```python
from build123d import *

# Parameters (mm, degrees)
CUT_EXTRUDE1_START = -2.5
CUT_EXTRUDE1_DEPTH = 2.5
SKETCH4_R          = 2.309401077
CUT_EXTRUDE2_DEPTH = 0.5
CUT_EXTRUDE2_TAPER = 45


with BuildPart() as part:
    # Sketch2 → Revolve1 (revolve)
    with BuildSketch(Plane(origin=(0, 0, 0), x_dir=(0, 0, -1), z_dir=(1, 0, 0))):
        Polygon((-9.25, 4.25), (-4.75, 4.25), (-4.5, 4), (-4.5, 2.5), (8.7, 2.5), (9.5, 1.7), (9.5, 0), (-9.5, 0), (-9.5, 4), align=None)
    revolve(axis=Axis((0, 0, -9.5), (0, 0, 1)))

    # Sketch3 → Cut-Extrude1 (cut)
    with BuildSketch(Plane.XY.offset(9.5).offset(CUT_EXTRUDE1_START)):
        Polygon((0, 2.309401077), (-2, 1.154700538), (-2, -1.154700538), (0, -2.309401077), (2, -1.154700538), (2, 1.154700538), align=None)
    extrude(amount=CUT_EXTRUDE1_DEPTH, mode=Mode.SUBTRACT)

    # Sketch4 → Cut-Extrude2 (cut)
    with BuildSketch(Plane.XY.offset(9.5)):
        Circle(SKETCH4_R)
    extrude(amount=-CUT_EXTRUDE2_DEPTH, taper=CUT_EXTRUDE2_TAPER, mode=Mode.SUBTRACT)


solid = part.part
```
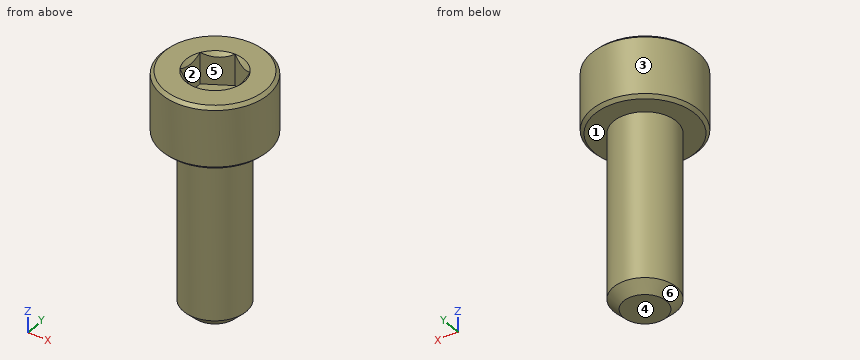
Part model, mm, in its own coordinate system. Face numbers are marked on the shaded views. A direction names the side the tool comes from. Give positions to 0.01 mm unless a question says otherwise; leave off trailing zeros. Order: outer loops, then holes, each group sorted by start corner. A loop starts at its lowest first (then second) coordinate and runs counter-clockwise, first axis right, second up. Notation, with made-up numbers: M -38,35.5 L -7,35.5 A33 ccw -7,74.5 Z; hole C 3,-36.75 d6. An arc over 180 degrees is marked long. Use a Markdown table: item, result. Add a question column.
(1) Probe line 1 along Z through (x, y) = (-1.25, -2.25); line 2 along X through (y, z) = (1.5, -4.75); line 3 along Z through (x, y) = (-1.5, -0.5). List the from-to ranges inside material, lowest first. Write a range as [from, to].
(2) Drop flat-ended pins along their axis: P1, Ø1.5, axis at x = 1.5, y = -1.5, coming from the +Z side; P2, Ø1, axis at x = 2.5, z = 5.5, coming from the -Y side; P3, Ø1.2, axis at x = -1, y = 0, coming from the +Z side; P4, Ø1, axis at y = -2.5, z = 5.5, coming from the +X side. Give the stop position or say it passes through.
(3) Saw through at A-A, the plane y = 0. Give the cut face in (x, z), and give its area (3 significant figures).
(4) 3-axis set-ups, long thin cutter, end or side, ignore diameter. For the marked faces 1, 2 and 3: which of +Z, -Z, +X, -X, +Y, -Y reach the whole face in a straight line?
(5) Saw through at C-C, the plane z = 5.5. Give the cut face in (x, y).
(6) Saw through at B-B, the plane z = -8. Give the cut face in (x, y).
(7) Mould opens along Y. For the marked faces 4, 5 and 6 say: +Y half, -Y half, draft (parallel to the pull), parting line (faces both ways), or undercut.
Answer key:
| question | item | result |
|---|---|---|
| 1 | line 1 | [4.5, 9.5] |
| 1 | line 2 | [-2, 2] |
| 1 | line 3 | [-9.5, 7] |
| 2 | P1 | z = 9.5 |
| 2 | P2 | y = -3.75 |
| 2 | P3 | z = 7 |
| 2 | P4 | x = 3.75 |
| 3 | outline | M -4.25,4.75 L -4,4.5 L -2.5,4.5 L -2.5,-8.7 L -1.7,-9.5 L 1.7,-9.5 L 2.5,-8.7 L 2.5,4.5 L 4,4.5 L 4.25,4.75 L 4.25,9.25 L 4,9.5 L 2.31,9.5 L 2,9.19 L 2,7 L -2,7 L -2,9.19 L -2.31,9.5 L -4,9.5 L -4.25,9.25 Z |
| 3 | area | 102 mm^2 |
| 4 | face 1 | -Z |
| 4 | face 2 | +Z |
| 4 | face 3 | +Z, -Z |
| 5 | outline | C 0,0 d8.5 |
| 6 | outline | C 0,0 d5 |
| 7 | face 4 | draft |
| 7 | face 5 | undercut |
| 7 | face 6 | parting line |
